Read the model definition and answer for the solid it produces. Units are mm, in the model's axes. Coordinates: 2 decimals unless noted, no trailing zeros. Order: outer loops, then holes, each group sorted by start corner. A loop starts at its lowest first (then second) coordinate and runs counter-clockwise, first axis right, second up. Notation, with made-up numbers: (-38.75, 24) -> (-18.75, 24) arc R26 ccw to (-18.75, 63) -> close; hole circle Ø6 at (-10, 83). An arc over 180 degrees is marked (long way). Answer in a Markdown table with one row per item.
from build123d import *

# Parameters (mm, degrees)
F0_R     = 0.48
F1_DEPTH = 7.6
F2_R     = 0.981
F2_R_2   = 0.48
F3_DEPTH = 2.8
F6_SCALE = 3


with BuildPart() as f1:
    # F0 (on Top) → F1 (new body)
    with BuildSketch(Plane.XY):
        Circle(F0_R)
    extrude(amount=F1_DEPTH)

    # F2 (on face) → F3 (join)
    with BuildSketch(Plane.XY.offset(7.6)):
        Circle(F2_R)
        Circle(F2_R_2, mode=Mode.SUBTRACT)
        Circle(F2_R_2)
    extrude(amount=F3_DEPTH)

    # F4 (on Front) → F5 (revolve)
    with BuildSketch(Plane.XZ):
        with BuildLine():
            Line((0, 10.4), (1, 10.4))
            ThreePointArc((1, 10.4), (0.7071067812, 11.1071067812), (0, 11.4))
            Line((0, 11.4), (0, 10.4))
        make_face()
    revolve(axis=Axis((0, 0, 7.5), (0, 0, 1)))


with BuildPart() as f1_1:
    # F6: moved
    add(f1.part.scale(F6_SCALE))


solid = f1_1.part
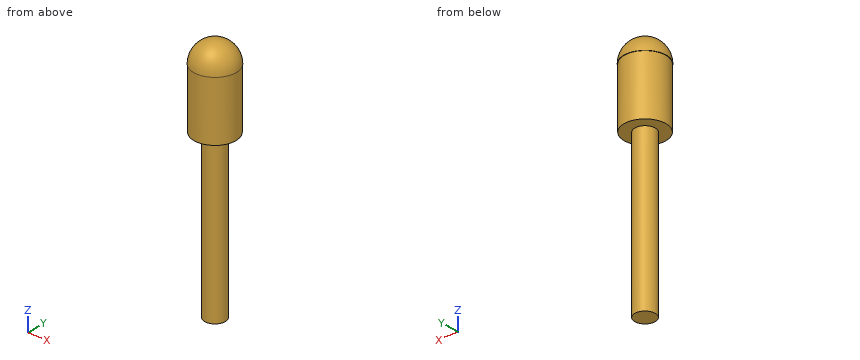
Q1. The part is cut by section D-D (x = 2.25). Write down the section's boundary in (y, z).
Outcome:
| item | result |
|---|---|
| outline | (-1.98, 31.2) -> (-1.9, 31.2) -> (-1.9, 22.8) -> (1.9, 22.8) -> (1.9, 31.2) -> (1.98, 31.2) arc R1.98 ccw to start |
Q2. Consider line 1 (X direction, y = -0.1, z = 7.5); line 2 (X direction, y = -0.15, z = 28.5); line 3 (Z direction, x = -0.75, y = 2.2). Determine where each line is inside the solid, lowest interval first.
Outcome:
| item | result |
|---|---|
| line 1 | -1.44 to 1.44 |
| line 2 | -2.94 to 2.94 |
| line 3 | 22.8 to 33.1 |
Q3. The part is cut by section C-C (z = 27). Write down the section's boundary in (x, y), then the cut area to 3 significant figures.
Outcome:
| item | result |
|---|---|
| outline | circle Ø5.89 at (0, 0) |
| area | 27.2 mm² |
Q4. The part is cut by section A-A (y = 0). Write down the section's boundary in (x, z).
Outcome:
| item | result |
|---|---|
| outline | (-3, 31.2) -> (-2.94, 31.2) -> (-2.94, 22.8) -> (-1.44, 22.8) -> (-1.44, 0) -> (1.44, 0) -> (1.44, 22.8) -> (2.94, 22.8) -> (2.94, 31.2) -> (3, 31.2) arc R3 ccw to start |
Q5. Given pin 1 (2 mm diameter, centred on x = -2, y = 0.5, fed in from +Z); pin 2 (1.8 mm diameter, centred on x = -0.5, y = 0, fed in from -Z); pin 3 (1 mm diameter, centred on y = -0.5, z = 16.5, fed in from +X), each flat-ended and moving along its own axis, determine where each tip first touches the part or whether it passes through.
Outcome:
| item | result |
|---|---|
| pin 1 | z = 34.01 |
| pin 2 | z = 0 |
| pin 3 | x = 1.44 |
